from build123d import *

# Parameters (mm, degrees)
AUFSATZ_LINEAR_AUSTRAGEN2_DEPTH   = 10
AUFSATZ_LINEAR_AUSTRAGEN2_2_DEPTH = 10
AUFSATZ_LINEAR_AUSTRAGEN3_DEPTH   = 10


with BuildPart() as part:
    # Skizze1 → Aufsatz-Linear austragen2 (new body)
    with BuildSketch(Plane.XY):
        Polygon((-10, 5.9), (0, 5.9), (30, 5.9), (54.574561329, 23.107293091), (62.766081772, 28.843057454), (57.030317408, 37.034577897), (26.847012111, 15.9), (-10, 15.9), align=None)
    extrude(amount=AUFSATZ_LINEAR_AUSTRAGEN2_DEPTH)



with BuildPart() as body_2:
    # Skizze1 → Aufsatz-Linear austragen2 2 (new body)
    with BuildSketch(Plane.XY):
        Polygon((31.860262854, 0), (0, 0), (-10, 0), (-10, -10), (35.013250743, -10), (71.88594711, 15.81853995), (66.150182746, 24.010060393), (57.958662303, 18.274296029), align=None)
    extrude(amount=AUFSATZ_LINEAR_AUSTRAGEN2_2_DEPTH)


with BuildPart() as part_1:
    add(part.part)

    add(body_2.part)  # Aufsatz-Linear austragen3 merges body 2
    # Skizze2 → Aufsatz-Linear austragen3 (add)
    with BuildSketch(Plane(origin=(0, 0, 0), x_dir=(-1, 0, 0), z_dir=(0, 0, -1))):
        Polygon((10, 15.9), (-26.847012111, 15.9), (-30, 5.9), (10, 5.9), align=None)
        Polygon((10, 5.9), (-30, 5.9), (-35.013250743, -10), (10, -10), align=None)
        Polygon((-30, 5.9), (-62.766081772, 28.843057454), (-71.88594711, 15.81853995), (-35.013250743, -10), align=None)
        Polygon((-26.847012111, 15.9), (-57.030317408, 37.034577897), (-62.766081772, 28.843057454), (-30, 5.9), align=None)
    extrude(amount=AUFSATZ_LINEAR_AUSTRAGEN3_DEPTH)


solid = part_1.part
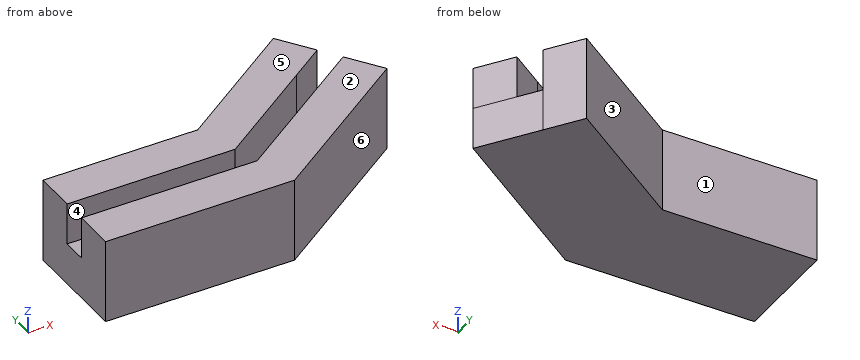
Here's how the part is built. I have some questions about the finished solid (model axes, mm). Face numbers are marked on the shaded views. A direction names the side the tool comes from. Give positions to 0.01 mm unless a question says otherwise; leave off trailing zeros. Order: outer loops, then holes, each group sorted by start corner. A loop starts at its lowest first (then second) coordinate and runs counter-clockwise, first axis right, second up. Notation, with made-up numbers: (0.25, 66) -> (59.25, 66) arc R18 cw to (59.25, 81) -> close; hole circle Ø7 at (1.5, 36). An arc over 180 degrees is marked (long way). Use a Markdown table: item, result. Add a question column.
Item 1: Imagine slicing it at C-C on y = 14.5. Please give me the cut outline in (x, z).
Item 2: Imagine slicing it at A-A on z = 3.5. Please give me the cut outline in (x, y), plus the area to 3 significant figures.
Item 3: I need wall thicknesses on line 1 (Y direction, x = 18, z = 7.5); line 2 (Y direction, x = 10, z = -9); line 3 (Y direction, x = 57, z = 5.5). Which ranges of each line are inside material? Lowest first, please.
Item 4: Imagine slicing it at B-B on x = 4.5. Please give me the cut outline in (y, z), plus the area to 3 significant figures.
Item 5: Imagine slicing it at D-D on y = 4. Please give me the cut outline in (x, z).
Item 6: Will these pins go through, and if not, where does the flat tip stop? pin 1 (1.5 mm diameter, centred on x = 40, z = 3.5, fed in from -Y); pin 2 (8 mm diameter, centred on y = 30.5, z = 1.5, fed in from +X); pin 3 (3 mm diameter, centred on x = 49, z = -5.5, fed in from +Y); pin 4 (6 mm diameter, centred on x = 18.5, y = 5.5, fed in from +Z).
Item 7: If we mould it in two halves opening along Y, with no side actions, what happens to the marked faces 3, 4, 5 and 6? For each: pulls with the +Y half, pulls with the -Y half, needs draft (parallel to the pull), parting line crosses it, or undercut.
Item 8: For the marked faces 1 and 2, which set-ups out of +Z, -Z, +X, -X, +Y, -Y let a thin tool reach every point of the face, with its end or its side?
Data:
| question | item | result |
|---|---|---|
| 1 | outline | (-10, -10) -> (70, -10) -> (70, 10) -> (52.57, 10) -> (52.57, 0) -> (42.28, 0) -> (42.28, 10) -> (-10, 10) -> close |
| 2 | outline | (-10, -10) -> (35.01, -10) -> (71.89, 15.82) -> (66.15, 24.01) -> (31.86, 0) -> (-10, 0) -> close; (-10, 5.9) -> (30, 5.9) -> (62.77, 28.84) -> (57.03, 37.03) -> (26.85, 15.9) -> (-10, 15.9) -> close |
| 2 | area | 1,640 mm² |
| 3 | line 1 | y = -10 to 0, 5.9 to 15.9 |
| 3 | line 2 | y = -10 to 15.9 |
| 3 | line 3 | y = 5.4 to 17.6, 24.81 to 37.01 |
| 4 | outline | (-10, -10) -> (15.9, -10) -> (15.9, 10) -> (5.9, 10) -> (5.9, 0) -> (0, 0) -> (0, 10) -> (-10, 10) -> close |
| 4 | area | 459 mm² |
| 5 | outline | (-10, -10) -> (55.01, -10) -> (55.01, 10) -> (37.57, 10) -> (37.57, 0) -> (-10, 0) -> close |
| 6 | pin 1 | stops at y = -7.03 |
| 6 | pin 2 | stops at x = 64.2 |
| 6 | pin 3 | stops at y = 32.46 |
| 6 | pin 4 | stops at z = 10 |
| 7 | face 3 | pulls with the +Y half |
| 7 | face 4 | undercut |
| 7 | face 5 | needs draft |
| 7 | face 6 | pulls with the -Y half |
| 8 | face 1 | +Z, -Z, -X, +Y |
| 8 | face 2 | +Z, +X, -X, +Y, -Y |
